Input: part model. Units: mm. Frame: model coordinates. A direction names the side the tool comes from. Round coordinates to 2 decimals unless told otherwise and drop trailing zeros. Loops run counter-clockwise (first coordinate to the right, second up) from the corner with the lowest first, then second, coordinate; pieces in that order, holes last. Notation, with made-up numbers: (22, 61) - (42, 61) arc R25 cw to (42, 87) - close; hole circle Ø7 at (3.25, 8). An arc over 180 degrees is marked (long way). Use CSV: the item, a comma, the result in double quotes. Start each with the question number.
1. Cut plane D-D (z = 26.25). Return loops of the section in (x, y), and give its area (3 significant figures).
2. Material intervals for probe 1 along X at (y, z) = (8.05, 3.5); probe 2 along X at (y, z) = (8.1, 6.75); probe 3 along X at (y, z) = (8.3, 1.5), sorted ascending. Write a range as from..to.
3. Access query for faces 1 (the flat face through (-19, 6.402, 14)), 2 (the flat face through (-30.346, 9, 16)), 3 (the flat face through (-7.346, 9, 16)). Directions: +Z, -Z, +X, -X, +Y, -Y. A direction counts if a zero-diameter tool reaches every point of the face in a straight line with its end or side. Return the directions, or none.
4. Pin query (flat end, axial travel): P1, Ø1.8, axis at x = -35.5, y = 8.5, coming from the +Z side; P2, Ø2, axis at y = 8, z = 24.5, coming from the +X side. Return the tip coordinate at first contact, or that it passes through.
5. Cut plane A-A (y = 11.7). Return loops of the section in (x, z), and give its area (3 significant figures).
6. Cut plane C-C (z = 3). Return loops of the section in (x, y), and give its area (3 significant figures).
7. Cut plane B-B (y = 8.45). Return loops of the section in (x, z), and give its area (3 significant figures).
8. Pull-direction query (X, two-part tool) for faces 4 (the cylindrical face through (-5.536, 8.489, 2.028)), 5 (the cylindrical face through (-31.915, 9.852, 2.028)), 6 (the flat face through (-37.346, 9, 2)), 7 (the flat face through (-2, 9, 4)); classes: +X half, -X half, draft (parallel to the pull), parting line (faces both ways), or undercut.
```python
from build123d import *

# Parameters (mm, degrees)
CROQUIS1_W              = 37
CROQUIS1_H              = 10
SALIENTE_EXTRUIR1_DEPTH = 25
CROQUIS2_W              = 37
CROQUIS2_H              = 6
CORTAR_EXTRUIR1_DEPTH   = 21
CROQUIS4_R              = 1.5
CORTAR_EXTRUIR2_DEPTH   = 4
CROQUIS6_W              = 37
CROQUIS6_H              = 4
CORTAR_EXTRUIR3_DEPTH   = 4
CROQUIS8_W              = 23
CROQUIS8_H              = 6
SALIENTE_EXTRUIR2_DEPTH = 25


with BuildPart() as part:
    # Croquis1 → Saliente-Extruir1 (new body)
    with BuildSketch(Plane.XY):
        with Locations((-18.845794393, 11.401869159)):
            Rectangle(CROQUIS1_W, CROQUIS1_H)
    extrude(amount=SALIENTE_EXTRUIR1_DEPTH)

    # Croquis2 → Cortar-Extruir1 (cut)
    with BuildSketch(Plane.XY.offset(25)):
        with Locations((-18.845794393, 9.401869159)):
            Rectangle(CROQUIS2_W, CROQUIS2_H)
    extrude(amount=-CORTAR_EXTRUIR1_DEPTH, mode=Mode.SUBTRACT)

    # Croquis4 → Cortar-Extruir2 (cut)
    with BuildSketch(Plane.XY.offset(4)):
        with Locations((-33.345794393, 9.401869159)):
            Circle(CROQUIS4_R)
        with Locations((-4.345794393, 9.401869159)):
            Circle(CROQUIS4_R)
    extrude(amount=-CORTAR_EXTRUIR2_DEPTH, mode=Mode.SUBTRACT)

    # Croquis6 → Cortar-Extruir3 (cut)
    with BuildSketch(Plane(origin=(0, 0, 0), x_dir=(-1, 0, 0), z_dir=(0, 0, -1))):
        with Locations((18.845794393, 14.401869159)):
            Rectangle(CROQUIS6_W, CROQUIS6_H)
    extrude(amount=-CORTAR_EXTRUIR3_DEPTH, mode=Mode.SUBTRACT)


with BuildPart() as cortar_extruir3_kept_piece:
    # of the separate pieces the step leaves, the one the design keeps (cortar_extruir3_pieces_kept)
    add(part.part.solids().sort_by_distance((-37.345794393, 6.401869159, 0))[0])

    # Croquis8 → Saliente-Extruir2 (add)
    with BuildSketch(Plane.XY.offset(4)):
        with Locations((-18.845794393, 9.401869159)):
            Rectangle(CROQUIS8_W, CROQUIS8_H)
    extrude(amount=SALIENTE_EXTRUIR2_DEPTH)


solid = cortar_extruir3_kept_piece.part
```
Established:
1,outline,"(-30.35, 6.4) - (-7.35, 6.4) - (-7.35, 12.4) - (-30.35, 12.4) - close"
1,area,"138 mm2"
2,probe 1,"x = -37.35..-34, -32.7..-5, -3.7..-0.35"
2,probe 2,"x = -30.35..-7.35"
2,probe 3,"x = -37.35..-34.36, -32.33..-5.36, -3.33..-0.35"
3,face 1,"+Z, -Z, +X, -X, -Y"
3,face 2,"+Z, -X, +Y, -Y"
3,face 3,"+Z, +X, +Y, -Y"
4,P1,"stops at z = 4"
4,P2,"stops at x = -7.35"
5,outline,"(-37.35, 0) - (-0.35, 0) - (-0.35, 4) - (-7.35, 4) - (-7.35, 29) - (-30.35, 29) - (-30.35, 4) - (-37.35, 4) - close"
5,area,"723 mm2"
6,outline,"(-37.35, 6.4) - (-0.35, 6.4) - (-0.35, 12.4) - (-37.35, 12.4) - close; hole circle Ø3 at (-33.35, 9.4); hole circle Ø3 at (-4.35, 9.4)"
6,area,"208 mm2"
7,outline,"(-37.35, 0) - (-34.51, 0) - (-34.51, 4) - (-37.35, 4) - close; (-32.19, 0) - (-5.51, 0) - (-5.51, 4) - (-7.35, 4) - (-7.35, 29) - (-30.35, 29) - (-30.35, 4) - (-32.19, 4) - close; (-3.19, 0) - (-0.35, 0) - (-0.35, 4) - (-3.19, 4) - close"
7,area,"704 mm2"
8,face 4,"undercut"
8,face 5,"undercut"
8,face 6,"-X half"
8,face 7,"draft"
